CAD build for the part. Positions are in the model's coordinates, mm. A direction names the side the tool comes from. Give positions to 0.01 mm unless a question says otherwise; leave off trailing zeros.
Item 1: Which spindle directions (+Z, -Z, +X, -X, +Y, -Y) get a long thin tool onto all of the face, cutting with end or side? Do faces 5 (the cylindrical face through (13.052, 0.086, 73.77)), 6 (the flat face through (-0.196, 5.472, 72.656)), 7 (the cylindrical face through (-0.9, 4.27, 6.61)), 8 (the flat face through (-0.025, 10.77, 5.715)), 9 (the flat face through (7.01, -1.97, 39.18)). Say none if no direction does.
Item 2: Saw through at A-A on x = -1. Give the number of separate pieces and of enclosed holes in the cut face, plus the area to 3 significant figures.
Item 3: Mould opens along X. For faces 1 (the flat face through (-0.2, -4.46, 71.87)), 2 (the flat face through (12.08, -2.03, 39.9)), 3 (the flat face through (-7.01, -1.97, 39.18)), 4 (the flat face through (0, 9, 0)) say: released by +X, released by -X, zero draft, split by the parting line, or undercut.
Item 4: Drop flat-ended pins along their axis: P1, Ø1, axis at x = 6, y = -3, coming from the -Z side; P2, Ø5, axis at y = 8, z = 58, coming from the +X side; P3, Ø8, axis at y = 10, z = 58.5, coming from the -X side. Give the stop position or say it passes through.
Item 5: Probe probe 1 along X at (y, z) = (-1.75, 70); probe 2 along X at (y, z) = (1.75, 11.5); probe 3 along Y at (x, z) = (-15, 74). List the from-to ranges inside material, lowest first.
from build123d import *

# Parameters (mm, degrees)
SKETCH3_R          = 1.95
CUT_EXTRUDE1_DEPTH = 20
SKETCH4_R          = 1.95
CUT_EXTRUDE2_DEPTH = 10
CUT_EXTRUDE3_DEPTH = 83.297374679
CHAMFER1_SIZE      = 2
CHAMFER1_SIZE_2    = 1.973894665
CHAMFER1_SIZE_3    = 2.02716926


with BuildPart() as part:
    # Loft1: read off the stored shape, not the designer's step
    # Loft1: loft between two sections, ruled curve by curve
    loft1_from = [
        Edge.make_line((-20, 6, 78.7), (20, 6, 78.7)),
        Edge.make_line((20, 6, 78.7), (20, -6, 78.7)),
        Edge.make_line((20, -6, 78.7), (-20, -6, 78.7)),
        Edge.make_line((-20, -6, 78.7), (-20, 6, 78.7)),
    ]
    loft1_to = [
        Edge.make_line((-6, 12, 0), (6, 12, 0)),
        Edge.make_line((6, 12, 0), (6, 0, 0)),
        Edge.make_line((6, 0, 0), (-6, 0, 0)),
        Edge.make_line((-6, 0, 0), (-6, 12, 0)),
    ]
    loft1 = Solid(Shell([*[Face.make_surface_from_curves(loft1_from[k], loft1_to[k]) for k in range(4)], Face(Wire(loft1_from)), Face(Wire(loft1_to))]))
    add(loft1)

    # Sketch3 → Cut-Extrude1 (cut)
    with BuildSketch(Plane(origin=(0, 0, 0), x_dir=(-1, 0, 0), z_dir=(0, 0, -1))):
        with Locations((0, 6)):
            Circle(SKETCH3_R)
    extrude(amount=-CUT_EXTRUDE1_DEPTH, mode=Mode.SUBTRACT)

    # Sketch4 → Cut-Extrude2 (cut)
    with BuildSketch(Plane.XY.offset(78.7)):
        with Locations((15, 0)):
            Circle(SKETCH4_R)
        with Locations((-15, 0)):
            Circle(SKETCH4_R)
    extrude(amount=-CUT_EXTRUDE2_DEPTH, mode=Mode.SUBTRACT)

    # Sketch5 → Cut-Extrude3 (cut, through all)
    with BuildSketch(Plane(origin=(0, 11.930654655, 0.90957977), x_dir=(1, 0, 0), z_dir=(0, 0.9971064242500265, 0.07601827885006555))):
        Polygon((-0.132366824, -6.087780654), (-11.649103048, -71.016165915), (11.649103048, -71.016165915), (0.132366824, -6.087780654), align=None)
    extrude(amount=-CUT_EXTRUDE3_DEPTH, mode=Mode.SUBTRACT)

    # Chamfer1
    # the kernel refuses this chamfer: 2.02716926, 2, 1.973894665 mm, written as the material it takes off along each edge
    with BuildSketch(Plane(origin=(-16.792469024, -5.398526703, 70.81067526), x_dir=(0, 0.997106424250026, 0.07601827885007145), z_dir=(1, 0, 0))) as chamfer1_piece_1_section:
        Polygon((CHAMFER1_SIZE, 0), (0, CHAMFER1_SIZE), (0, 0), align=None)
    chamfer1_piece_1 = extrude(amount=33.584938049, mode=Mode.PRIVATE)
    chamfer1_piece_1 = split(chamfer1_piece_1, bisect_by=Plane(origin=(-15.283859564, -6.946592893, 70.961020054), z_dir=(0.6962389816670421, -0.7144486731771176, 0.06938568874556392)), keep=Keep.TOP, mode=Mode.PRIVATE)
    chamfer1_piece_1 = split(chamfer1_piece_1, bisect_by=Plane(origin=(-2.020822768, 9.759462645, 69.338564567), z_dir=(-0.6962389816670431, -0.7144486731771169, 0.0693856887455642)), keep=Keep.TOP, mode=Mode.PRIVATE)
    add(chamfer1_piece_1, mode=Mode.SUBTRACT)
    with BuildSketch(Plane(origin=(-12.547391008, -5.783507257, 75.86033686), x_dir=(0, 0.9971064242500265, 0.07601827885006568), z_dir=(0.1746498234023745, 0.0748499243153034, -0.9817815072690628))) as chamfer1_piece_2_section:
        Polygon((CHAMFER1_SIZE, 0), (0, -CHAMFER1_SIZE), (0, 0), align=None)
    chamfer1_piece_2 = extrude(amount=76.22860352, mode=Mode.PRIVATE)
    chamfer1_piece_2 = split(chamfer1_piece_2, bisect_by=Plane(origin=(-12.547391008, 32.845065601, 42.704525209), z_dir=(0, -0.7588137546208746, 0.6513076736828541)), keep=Keep.TOP, mode=Mode.PRIVATE)
    chamfer1_piece_2 = split(chamfer1_piece_2, bisect_by=Plane(origin=(-12.547391008, -7.194759635, 74.216140486), z_dir=(0, -0.6513076736828518, -0.7588137546208766)), keep=Keep.TOP, mode=Mode.PRIVATE)
    add(chamfer1_piece_2, mode=Mode.SUBTRACT)
    with BuildSketch(Plane(origin=(12.547391008, -5.783507257, 75.86033686), x_dir=(1.43368408515118e-15, 0.9971064242500265, 0.07601827885006535), z_dir=(-0.17464982340237462, 0.07484992431530343, -0.9817815072690628))) as chamfer1_piece_3_section:
        Polygon((CHAMFER1_SIZE, 0), (0, CHAMFER1_SIZE), (0, 0), align=None)
    chamfer1_piece_3 = extrude(amount=76.22860352, mode=Mode.PRIVATE)
    chamfer1_piece_3 = split(chamfer1_piece_3, bisect_by=Plane(origin=(12.547391008, 32.845065601, 42.704525209), z_dir=(0, -0.7588137546208746, 0.6513076736828541)), keep=Keep.TOP, mode=Mode.PRIVATE)
    chamfer1_piece_3 = split(chamfer1_piece_3, bisect_by=Plane(origin=(12.547391008, -7.194759635, 74.216140486), z_dir=(0, -0.6513076736828518, -0.7588137546208766)), keep=Keep.TOP, mode=Mode.PRIVATE)
    add(chamfer1_piece_3, mode=Mode.SUBTRACT)
    with BuildSketch(Plane(origin=(-16.792469024, 6.532127952, 71.72025503), x_dir=(0, -0.07601827885006952, 0.9971064242500263), z_dir=(1, 0, 0))) as chamfer1_piece_4_section:
        Polygon((CHAMFER1_SIZE, 0), (0, CHAMFER1_SIZE), (0, 0), align=None)
    chamfer1_piece_4 = extrude(amount=33.584938049, mode=Mode.PRIVATE)
    chamfer1_piece_4 = split(chamfer1_piece_4, bisect_by=Plane(origin=(-15.283859564, 8.039510514, 72.103543821), z_dir=(0.6962389816670405, 0.6956727551266126, 0.1768917696835863)), keep=Keep.TOP, mode=Mode.PRIVATE)
    chamfer1_piece_4 = split(chamfer1_piece_4, bisect_by=Plane(origin=(-2.020822768, -8.227505047, 67.967258263), z_dir=(-0.6962389816670409, 0.6956727551266121, 0.17689176968358636)), keep=Keep.TOP, mode=Mode.PRIVATE)
    add(chamfer1_piece_4, mode=Mode.SUBTRACT)
    with BuildSketch(Plane(origin=(12.547391008, 6.147147398, 76.769916631), x_dir=(0.9846306105263636, 0.013276578976513069, -0.17414446090864058), z_dir=(-0.17464982340237462, 0.07484992431530339, -0.9817815072690629))) as chamfer1_piece_5_section:
        Polygon((CHAMFER1_SIZE, 0), (0, CHAMFER1_SIZE), (0, 0), align=None)
    chamfer1_piece_5 = extrude(amount=76.22860352, mode=Mode.PRIVATE)
    chamfer1_piece_5 = split(chamfer1_piece_5, bisect_by=Plane(origin=(12.547391008, 7.791343772, 75.358664253), z_dir=(0, 0.7588137546208767, -0.6513076736828517)), keep=Keep.TOP, mode=Mode.PRIVATE)
    chamfer1_piece_5 = split(chamfer1_piece_5, bisect_by=Plane(origin=(12.547391008, -27.008664253, 38.141343772), z_dir=(0, 0.6513076736828546, 0.7588137546208742)), keep=Keep.TOP, mode=Mode.PRIVATE)
    add(chamfer1_piece_5, mode=Mode.SUBTRACT)
    with BuildSketch(Plane(origin=(0.765921135, 11.852852602, 1.930083369), x_dir=(-0.9846306105263636, 0.013276578976513059, -0.17414446090864047), z_dir=(-0.1746498234023745, -0.07484992431530339, 0.9817815072690629))) as chamfer1_piece_6_section:
        Polygon((CHAMFER1_SIZE, 0), (0, CHAMFER1_SIZE), (0, 0), align=None)
    chamfer1_piece_6 = extrude(amount=76.22860352, mode=Mode.PRIVATE)
    chamfer1_piece_6 = split(chamfer1_piece_6, bisect_by=Plane(origin=(0.765921135, -26.775720256, 35.08589502), z_dir=(0, 0.7588137546208767, -0.6513076736828517)), keep=Keep.TOP, mode=Mode.PRIVATE)
    chamfer1_piece_6 = split(chamfer1_piece_6, bisect_by=Plane(origin=(0.765921135, 13.26410498, 3.574279744), z_dir=(0, 0.6513076736828546, 0.7588137546208742)), keep=Keep.TOP, mode=Mode.PRIVATE)
    add(chamfer1_piece_6, mode=Mode.SUBTRACT)
    with BuildSketch(Plane(origin=(-5.2757328, -0.462782607, 6.070165199), x_dir=(0, 0.0760182788500654, -0.9971064242500265), z_dir=(1, 0, 0))) as chamfer1_piece_7_section:
        Polygon((CHAMFER1_SIZE, 0), (0, CHAMFER1_SIZE), (0, 0), align=None)
    chamfer1_piece_7 = extrude(amount=10.5514656, mode=Mode.PRIVATE)
    chamfer1_piece_7 = split(chamfer1_piece_7, bisect_by=Plane(origin=(-3.767123339, -2.010848797, 6.220509994), z_dir=(0.6962389816670421, -0.7144486731771176, 0.06938568874556392)), keep=Keep.TOP, mode=Mode.PRIVATE)
    chamfer1_piece_7 = split(chamfer1_piece_7, bisect_by=Plane(origin=(-1.669532821, 3.237735258, 5.710779017), z_dir=(-0.6962389816670431, -0.7144486731771169, 0.0693856887455642)), keep=Keep.TOP, mode=Mode.PRIVATE)
    add(chamfer1_piece_7, mode=Mode.SUBTRACT)
    with BuildSketch(Plane(origin=(5.2757328, 11.467872048, 6.97974497), x_dir=(0, 0.0760182788500616, -0.9971064242500267), z_dir=(-1, 0, 0))) as chamfer1_piece_8_section:
        Polygon((CHAMFER1_SIZE, 0), (0, CHAMFER1_SIZE), (0, 0), align=None)
    chamfer1_piece_8 = extrude(amount=10.5514656, mode=Mode.PRIVATE)
    chamfer1_piece_8 = split(chamfer1_piece_8, bisect_by=Plane(origin=(1.669532821, 7.864604864, 6.063526383), z_dir=(0.6962389816670405, 0.6956727551266126, 0.1768917696835863)), keep=Keep.TOP, mode=Mode.PRIVATE)
    chamfer1_piece_8 = split(chamfer1_piece_8, bisect_by=Plane(origin=(3.767123339, 12.97525461, 7.36303376), z_dir=(-0.6962389816670409, 0.6956727551266121, 0.17689176968358636)), keep=Keep.TOP, mode=Mode.PRIVATE)
    add(chamfer1_piece_8, mode=Mode.SUBTRACT)
    with BuildSketch(Plane(origin=(20.898287959, 5.615019446, 83.7496616), x_dir=(-0.9846306105263637, -0.013276578976516254, 0.17414446090864033), z_dir=(-0.17464982340237456, 0.07484992431530338, -0.9817815072690627))) as chamfer1_piece_9:
        Polygon((CHAMFER1_SIZE, 0), (CHAMFER1_SIZE_2 * 0.0133139270738, -CHAMFER1_SIZE_2 * 0.999911365776), (0, 0), align=None)
    extrude(amount=90.447133647, mode=Mode.SUBTRACT)
    with BuildSketch(Plane(origin=(-20.898287959, 5.615019446, 83.7496616), x_dir=(0.9846306105263636, -0.013276578976516233, 0.17414446090864033), z_dir=(0.17464982340237456, 0.07484992431530338, -0.9817815072690627))) as chamfer1_piece_10:
        Polygon((CHAMFER1_SIZE_2, 0), (CHAMFER1_SIZE * 0.0133139270733, CHAMFER1_SIZE * 0.999911365745), (0, 0), align=None)
    extrude(amount=90.447133647, mode=Mode.SUBTRACT)
    with BuildSketch(Plane(origin=(-20.910812675, -6.390348289, 83.820068396), x_dir=(-0.013109300142731543, 0.9971948098691615, 0.07369299437378306), z_dir=(0.17464982340237456, 0.07484992431530338, -0.9817815072690627))) as chamfer1_piece_11:
        Polygon((CHAMFER1_SIZE_3, 0), (-CHAMFER1_SIZE * 0.0133139270733, CHAMFER1_SIZE * 0.999911365745), (0, 0), align=None)
    extrude(amount=90.590560255, mode=Mode.SUBTRACT)
    with BuildSketch(Plane(origin=(20.910812675, -6.390348289, 83.820068396), x_dir=(0.01310930014273147, 0.9971948098691616, 0.07369299437378309), z_dir=(-0.17464982340237456, 0.07484992431530338, -0.9817815072690627))) as chamfer1_piece_12:
        Polygon((CHAMFER1_SIZE, 0), (-CHAMFER1_SIZE_3 * 0.0133139270755, -CHAMFER1_SIZE_3 * 0.99991136591), (0, 0), align=None)
    extrude(amount=90.590560255, mode=Mode.SUBTRACT)


solid = part.part
Results below:
1. face 5: +Z
1. face 6: +Y
1. face 7: -Z
1. face 8: +Z, +Y
1. face 9: -Y
2. separate pieces: 3
2. enclosed holes: 0
2. area: 165 mm2
3. face 1: undercut
3. face 2: released by +X
3. face 3: undercut
3. face 4: zero draft
4. P1: stops at z = 70.96
4. P2: stops at x = 16.41
4. P3: stops at x = -15.96
5. probe 1: x = -18.45 to -15.86, -14.14 to -11.46, 11.46 to 14.14, 15.86 to 18.45
5. probe 2: x = -8.05 to -1.06, 1.06 to 8.05
5. probe 3: y = -5.64 to -1.95, 1.95 to 6.36
